from build123d import *

# Parameters (mm, degrees)
SKETCH1_R           = 11
BOSS_EXTRUDE1_DEPTH = 1
SKETCH2_R           = 5
BOSS_EXTRUDE2_DEPTH = 12
SKETCH3_R           = 3
CUT_EXTRUDE1_DEPTH  = 12
CUT_EXTRUDE2_REACH  = 21.647
SKETCH4_R           = 1.591156764


with BuildPart() as part:
    # Sketch1 → Boss-Extrude1 (new body)
    with BuildSketch(Plane(origin=(0, 0, 0), x_dir=(1, 0, 0), z_dir=(0, 1, 0))):
        with Locations(Location((0, 0, 0), (0, 0, 270))):
            Circle(SKETCH1_R)
    extrude(amount=BOSS_EXTRUDE1_DEPTH)

    # Sketch2 → Boss-Extrude2 (add)
    with BuildSketch(Plane(origin=(0, 1, 0), x_dir=(1, 0, 0), z_dir=(0, 1, 0))):
        with Locations(Location((0, 0, 0), (0, 0, 270))):
            Circle(SKETCH2_R)
    extrude(amount=BOSS_EXTRUDE2_DEPTH)

    # Sketch3 → Cut-Extrude1 (cut)
    with BuildSketch(Plane(origin=(0, 13, 0), x_dir=(1, 0, 0), z_dir=(0, 1, 0))):
        with Locations(Location((0, 0, 0), (0, 0, 270))):
            Circle(SKETCH3_R)
    extrude(amount=-CUT_EXTRUDE1_DEPTH, mode=Mode.SUBTRACT)

    # Sketch4 → Cut-Extrude2 (cut, up to next)
    with BuildSketch(Plane(origin=(0, 1, 0), x_dir=(1, 0, 0), z_dir=(0, 1, 0)), mode=Mode.PRIVATE) as cut_extrude2_sk1:
        with Locations(Location((5.355689552, 5.380973844, 0), (0, 0, 270))):
            Circle(SKETCH4_R)
    cut_extrude2_tool1 = extrude(cut_extrude2_sk1.sketch, amount=-CUT_EXTRUDE2_REACH, mode=Mode.PRIVATE) & part.part
    # Sketch4 → Cut-Extrude2 (cut, up to next)
    with BuildSketch(Plane(origin=(0, 1, 0), x_dir=(1, 0, 0), z_dir=(0, 1, 0)), mode=Mode.PRIVATE) as cut_extrude2_sk2:
        with Locations(Location((-5.42311433, 5.380973844, 0), (0, 0, 270))):
            Circle(SKETCH4_R)
    cut_extrude2_tool2 = extrude(cut_extrude2_sk2.sketch, amount=-CUT_EXTRUDE2_REACH, mode=Mode.PRIVATE) & part.part
    # Sketch4 → Cut-Extrude2 (cut, up to next)
    with BuildSketch(Plane(origin=(0, 1, 0), x_dir=(1, 0, 0), z_dir=(0, 1, 0)), mode=Mode.PRIVATE) as cut_extrude2_sk3:
        with Locations(Location((-5.42311433, -5.397830038, 0), (0, 0, 270))):
            Circle(SKETCH4_R)
    cut_extrude2_tool3 = extrude(cut_extrude2_sk3.sketch, amount=-CUT_EXTRUDE2_REACH, mode=Mode.PRIVATE) & part.part
    # Sketch4 → Cut-Extrude2 (cut, up to next)
    with BuildSketch(Plane(origin=(0, 1, 0), x_dir=(1, 0, 0), z_dir=(0, 1, 0)), mode=Mode.PRIVATE) as cut_extrude2_sk4:
        with Locations(Location((5.355689552, -5.397830038, 0), (0, 0, 270))):
            Circle(SKETCH4_R)
    cut_extrude2_tool4 = extrude(cut_extrude2_sk4.sketch, amount=-CUT_EXTRUDE2_REACH, mode=Mode.PRIVATE) & part.part
    add(cut_extrude2_tool1.solids().sort_by_distance((5.35569, 1, -5.380974))[0], mode=Mode.SUBTRACT)
    add(cut_extrude2_tool2.solids().sort_by_distance((-5.423114, 1, -5.380974))[0], mode=Mode.SUBTRACT)
    add(cut_extrude2_tool3.solids().sort_by_distance((-5.423114, 1, 5.39783))[0], mode=Mode.SUBTRACT)
    add(cut_extrude2_tool4.solids().sort_by_distance((5.35569, 1, 5.39783))[0], mode=Mode.SUBTRACT)


solid = part.part
Input: part model. Units: mm. Frame: model coordinates. A direction names the side the tool comes from. Coordinates: 2 decimals unless noted, no trailing zeros. Write each loop counter-clockwise with the first axis right and the second up, starting at its lowest first coordinate (ties: lowest second). Pieces come first, ordered by that corner, then holes. Notation, with made-up numbers: M 15.25,-35 L 46.25,-35 A26 ccw 46.25,-9 Z; hole C 20.5,58.5 d5. An arc over 180 degrees is marked long. Answer as a JSON object with one key per item and string values. Group by question number.
(1) Section A-A on x = -5.75. Output: boundary loops of the cut face in (y, z).
(2) Ray query, line 1 along Y through (x, z) = (1.5, -0.5); line 2 along Z through (x, y) = (-1, 4.5); line 3 along X through (y, z) = (10.75, 0). Return the intervals inside material, ascending. Write a range as [from, to].
(3) Section C-C on y = 3. Output: boundary loops of the cut face in (x, z), plus the area to 3 significant figures.
(4) Set-up query: faces 1 (the face through (0, 1, 0)), 2 (the face through (-4.95, 0.51, -3.86)). Return all of +Z, -Z, +X, -X, +Y, -Y with unobstructed straight access to the full face (end or side cutting, diameter ignored); none if empty.
(5) Contact query for flat-ended pins moving along their axis: P1, Ø6, axis at x = -2, y = 9.5, coming from the +Z side; P2, Ø2, axis at y = 9.5, z = -4, coming from the +X side; P3, Ø3, axis at y = 1.5, z = -4.5, coming from the +X side; P4, Ø2.5, axis at x = 5.36, z = -5.38, coming from the +Y side. Output: stop coordinate, or through.
(6) Section B-B on z = 0. Output: boundary loops of the cut face in (x, y), plus the area to 3 significant figures.
(7) Section D-D on z = 6. Output: boundary loops of the cut face in (x, y).
(8) Mould query, pull axis X, two halves, no side actions, for faces 3 (the face through (-3.3, 13, -0.1)), 4 (the face through (4.75, 0.51, -3.91)), 5 (the face through (-4.88, 6.92, -1.08)). Classes: pulls with the +X half, pulls with the -X half, needs draft (parallel to the pull), parting line crosses it, or undercut.
Result set:
{
 "1": {"outline": "M 0,-9.38 L 1,-9.38 L 1,-6.94 L 0,-6.94 Z; M 0,-3.82 L 1,-3.82 L 1,3.84 L 0,3.84 Z; M 0,6.96 L 1,6.96 L 1,9.38 L 0,9.38 Z"},
 "2": {"line 1": "y = [0, 1]", "line 2": "z = [-4.9, -2.83], [2.83, 4.9]", "line 3": "x = [-5, -3], [3, 5]"},
 "3": {"outline": "C 0,0 d10; hole C 0,0 d6", "area": "50.3 mm2"},
 "4": {"face 1": "+Y", "face 2": "+Y, -Y"},
 "5": {"P1": "stops at z = 5", "P2": "stops at x = 4", "P3": "stops at x = 10.56", "P4": "passes through"},
 "6": {"outline": "M -11,0 L 11,0 L 11,1 L 5,1 L 5,13 L 3,13 L 3,1 L -3,1 L -3,13 L -5,13 L -5,1 L -11,1 Z", "area": "70.0 mm2"},
 "7": {"outline": "M -9.22,0 L -6.9,0 L -6.9,1 L -9.22,1 Z; M -3.95,0 L 3.88,0 L 3.88,1 L -3.95,1 Z; M 6.83,0 L 9.22,0 L 9.22,1 L 6.83,1 Z"},
 "8": {"face 3": "needs draft", "face 4": "undercut", "face 5": "parting line crosses it"}
}
